from build123d import *

# Parameters (mm, degrees)
F0_R     = 11.0109
F0_R_2   = 3.175
F1_DEPTH = 6.35


with BuildPart() as f1:
    # F0 (on Front) → F1 (new body)
    with BuildSketch(Plane.XZ):
        with BuildLine():
            ThreePointArc((12.3733379566, 24.60625), (13.8006652431, 28.0521228931), (14.2875, 31.75))
            ThreePointArc((14.2875, 31.75), (10.1027881362, 41.8527881362), (0, 46.0375))
            ThreePointArc((0, 46.0375), (-10.1027881362, 41.8527881362), (-14.2875, 31.75))
            ThreePointArc((-14.2875, 31.75), (-13.8006652431, 28.0521228931), (-12.3733379566, 24.60625))
            ThreePointArc((-12.3733379566, 24.60625), (0, 17.4625), (12.3733379566, 24.60625))
        make_face()
        with Locations((0, 31.75)):
            Circle(F0_R, mode=Mode.SUBTRACT)
        with BuildLine():
            ThreePointArc((-14.2875, 31.75), (-10.1027881362, 41.8527881362), (0, 46.0375))
            ThreePointArc((0, 46.0375), (-20.8568006936, 40.269983922), (-35.7872332561, 24.60625))
            ThreePointArc((-35.7872332561, 24.60625), (-26.2265027578, 31.7569329924), (-14.2875, 31.75))
        make_face()
        with BuildLine():
            ThreePointArc((10.6471746219, 11.2874452221), (10.1786438017, 18.1194292121), (12.3733379566, 24.60625))
            ThreePointArc((12.3733379566, 24.60625), (0, 17.4625), (-12.3733379566, 24.60625))
            ThreePointArc((-12.3733379566, 24.60625), (-10.2077366082, 18.3335066447), (-10.5388292946, 11.7057230006))
            ThreePointArc((-10.5388292946, 11.7057230006), (-10.3260856779, 10.8481793102), (-10.2344309309, 9.9694071925))
            ThreePointArc((-10.2344309309, 9.9694071925), (0.1150101412, 14.2870370937), (10.3936009423, 9.8033522686))
            ThreePointArc((10.3936009423, 9.8033522686), (10.4762468955, 10.5529407036), (10.6471746219, 11.2874452221))
        make_face()
        with BuildLine():
            ThreePointArc((23.0855388403, 9.4834715128), (17.6469627848, 15.7677221756), (10.6471746219, 11.2874452221))
            ThreePointArc((10.6471746219, 11.2874452221), (11.3765560575, 9.1599013663), (12.3733379177, 7.1437500673))
            ThreePointArc((12.3733379177, 7.1437500673), (13.7532190864, 5.1015858399), (15.4068681354, 3.274032395))
            ThreePointArc((15.4068681354, 3.274032395), (20.7283724847, 4.5458830844), (23.0855388403, 9.4834715128))
        make_face()
        with Locations((16.7355388403, 9.4834715128)):
            Circle(F0_R_2, mode=Mode.SUBTRACT)
        with BuildLine():
            ThreePointArc((12.3733379177, 7.1437500673), (11.3765560575, 9.1599013663), (10.6471746219, 11.2874452221))
            ThreePointArc((10.6471746219, 11.2874452221), (10.4762468955, 10.5529407036), (10.3936009423, 9.8033522686))
            ThreePointArc((10.3936009423, 9.8033522686), (11.4608789903, 8.531172781), (12.3733379177, 7.1437500673))
        make_face()
        with BuildLine():
            ThreePointArc((-10.2344309309, 9.9694071925), (-10.3260856779, 10.8481793102), (-10.5388292946, 11.7057230006))
            ThreePointArc((-10.5388292946, 11.7057230006), (-11.2947124555, 9.359844254), (-12.3733379294, 7.1437500471))
            ThreePointArc((-12.3733379294, 7.1437500471), (-11.3918342591, 8.6231530466), (-10.2344309309, 9.9694071925))
        make_face()
        with BuildLine():
            ThreePointArc((-12.3733379294, 7.1437500471), (-11.2947124555, 9.359844254), (-10.5388292946, 11.7057230006))
            ThreePointArc((-10.5388292946, 11.7057230006), (-22.1188173057, 12.8583877354), (-15.0988016171, 3.57700109))
            ThreePointArc((-15.0988016171, 3.57700109), (-13.620985268, 5.2724359227), (-12.3733379294, 7.1437500471))
        make_face()
        with Locations((-16.5806966663, 9.7516660253)):
            Circle(F0_R_2, mode=Mode.SUBTRACT)
        with BuildLine():
            ThreePointArc((15.4068681354, 3.274032395), (13.7532190864, 5.1015858399), (12.3733379177, 7.1437500673))
            ThreePointArc((12.3733379177, 7.1437500673), (13.1637867029, 5.5540414017), (13.7509753549, 3.8785735832))
            ThreePointArc((13.7509753549, 3.8785735832), (14.5578417064, 3.5185628636), (15.4068681354, 3.274032395))
        make_face()
        with BuildLine():
            ThreePointArc((-13.686752578, 4.0994463185), (-13.1186518214, 5.6598260255), (-12.3733379294, 7.1437500471))
            ThreePointArc((-12.3733379294, 7.1437500471), (-13.620985268, 5.2724359227), (-15.0988016171, 3.57700109))
            ThreePointArc((-15.0988016171, 3.57700109), (-14.3772381817, 3.796225596), (-13.686752578, 4.0994463185))
        make_face()
        with BuildLine():
            ThreePointArc((-13.686752578, 4.0994463185), (-14.3772381817, 3.796225596), (-15.0988016171, 3.57700109))
            ThreePointArc((-15.0988016171, 3.57700109), (-20.7812079006, -0.2447504977), (-27.4963065702, -1.5875))
            ThreePointArc((-27.4963065702, -1.5875), (-17.393518434, -5.7722118638), (-13.2088065702, -15.875))
            ThreePointArc((-13.2088065702, -15.875), (-13.6956413271, -19.5728771069), (-15.1229686136, -23.01875))
            ThreePointArc((-15.1229686136, -23.01875), (-10.7734141907, -18.0069125403), (-4.8680388409, -14.9797553955))
            ThreePointArc((-4.8680388409, -14.9797553955), (-4.2317560285, -14.3667421738), (-3.5165444239, -13.8479807757))
            ThreePointArc((-3.5165444239, -13.8479807757), (-12.4304421386, -7.0439168429), (-13.686752578, 4.0994463185))
        make_face()
        with BuildLine():
            ThreePointArc((15.4068681354, 3.274032395), (14.5578417064, 3.5185628636), (13.7509753549, 3.8785735832))
            ThreePointArc((13.7509753549, 3.8785735832), (14.1527332454, 1.9577532873), (14.2875, 0))
            ThreePointArc((14.2875, 0), (11.2067738499, -8.8623290464), (3.2931516357, -13.9027985871))
            ThreePointArc((3.2931516357, -13.9027985871), (3.9009912862, -14.3491662996), (4.4516269953, -14.8644463122))
            ThreePointArc((4.4516269953, -14.8644463122), (10.6025640989, -17.8746787144), (15.1229686136, -23.01875))
            ThreePointArc((15.1229686136, -23.01875), (15.1229686136, -8.73125), (27.4963065702, -1.5875))
            ThreePointArc((27.4963065702, -1.5875), (20.9811507989, -0.3265941045), (15.4068681354, 3.274032395))
        make_face()
        with BuildLine():
            ThreePointArc((-13.2088065702, -15.875), (-17.393518434, -5.7722118638), (-27.4963065702, -1.5875))
            ThreePointArc((-27.4963065702, -1.5875), (-39.8696445267, -8.73125), (-39.8696445267, -23.01875))
            ThreePointArc((-39.8696445267, -23.01875), (-31.1941836771, -29.6756652431), (-20.3525565702, -28.2483379566))
            ThreePointArc((-20.3525565702, -28.2483379566), (-17.393518434, -25.9777881362), (-15.1229686136, -23.01875))
            ThreePointArc((-15.1229686136, -23.01875), (-13.6956413271, -19.5728771069), (-13.2088065702, -15.875))
        make_face()
        with Locations((-27.4963065702, -15.875)):
            Circle(F0_R, mode=Mode.SUBTRACT)
        with BuildLine():
            ThreePointArc((34.6400565702, -3.5016620434), (31.1941836771, -2.0743347569), (27.4963065702, -1.5875))
            ThreePointArc((27.4963065702, -1.5875), (15.1229686136, -8.73125), (15.1229686136, -23.01875))
            ThreePointArc((15.1229686136, -23.01875), (27.4963065702, -30.1625), (39.8696445267, -23.01875))
            ThreePointArc((39.8696445267, -23.01875), (41.2969718133, -19.5728771069), (41.7838065702, -15.875))
            ThreePointArc((41.7838065702, -15.875), (39.8696445267, -8.73125), (34.6400565702, -3.5016620434))
        make_face()
        with Locations((27.4963065702, -15.875)):
            Circle(F0_R, mode=Mode.SUBTRACT)
        with BuildLine():
            ThreePointArc((-5.5e-09, -14.2875), (-1.7719524453, -14.1771943903), (-3.5165444239, -13.8479807757))
            ThreePointArc((-3.5165444239, -13.8479807757), (-4.2317560285, -14.3667421738), (-4.8680388409, -14.9797553955))
            ThreePointArc((-4.8680388409, -14.9797553955), (-2.4585066475, -14.4614300385), (-5.5e-09, -14.2875))
        make_face()
        with BuildLine():
            ThreePointArc((-20.3525565702, -28.2483379566), (-31.1941836771, -29.6756652431), (-39.8696445267, -23.01875))
            ThreePointArc((-39.8696445267, -23.01875), (-24.4464287396, -38.1975112033), (-3.4160209638, -43.2957781309))
            ThreePointArc((-3.4160209638, -43.2957781309), (-14.3890593388, -38.5912841369), (-20.3525565702, -28.2483379566))
        make_face()
        with BuildLine():
            ThreePointArc((4.4516269953, -14.8644463122), (3.9009912862, -14.3491662996), (3.2931516357, -13.9027985871))
            ThreePointArc((3.2931516357, -13.9027985871), (1.6577728159, -14.1909987506), (-5.5e-09, -14.2875))
            ThreePointArc((-5.5e-09, -14.2875), (2.2444292093, -14.4323372312), (4.4516269953, -14.8644463122))
        make_face()
        with BuildLine():
            ThreePointArc((39.2032542199, 18.6895281309), (40.6155620966, 6.8343511445), (34.6400565702, -3.5016620434))
            ThreePointArc((34.6400565702, -3.5016620434), (39.8696445267, -8.73125), (41.7838065702, -15.875))
            ThreePointArc((41.7838065702, -15.875), (41.2969718133, -19.5728771069), (39.8696445267, -23.01875))
            ThreePointArc((39.8696445267, -23.01875), (45.3032294332, -2.0724727187), (39.2032542199, 18.6895281309))
        make_face()
        with BuildLine():
            ThreePointArc((4.4516269953, -14.8644463122), (2.2444292093, -14.4323372312), (-5.5e-09, -14.2875))
            ThreePointArc((-5.5e-09, -14.2875), (-2.4585066475, -14.4614300385), (-4.8680388409, -14.9797553955))
            ThreePointArc((-4.8680388409, -14.9797553955), (-2.4345023642, -25.1618271215), (6.195157826, -19.2351375381))
            ThreePointArc((6.195157826, -19.2351375381), (5.743190516, -16.8823284962), (4.4516269953, -14.8644463122))
        make_face()
        with Locations((-0.154842174, -19.2351375381)):
            Circle(F0_R_2, mode=Mode.SUBTRACT)
        with BuildLine():
            ThreePointArc((13.7509753549, 3.8785735832), (11.2108978898, 6.3528418048), (10.3936009423, 9.8033522686))
            ThreePointArc((10.3936009423, 9.8033522686), (0.1150101412, 14.2870370937), (-10.2344309309, 9.9694071925))
            ThreePointArc((-10.2344309309, 9.9694071925), (-10.2316303011, 9.8605526184), (-10.2306966663, 9.7516660253))
            ThreePointArc((-10.2306966663, 9.7516660253), (-11.1631767097, 6.4391175321), (-13.686752578, 4.0994463185))
            ThreePointArc((-13.686752578, 4.0994463185), (-12.4304421386, -7.0439168429), (-3.5165444239, -13.8479807757))
            ThreePointArc((-3.5165444239, -13.8479807757), (-0.1037265557, -12.8853432742), (3.2931516357, -13.9027985871))
            ThreePointArc((3.2931516357, -13.9027985871), (11.2067738499, -8.8623290464), (14.2875, 0))
            ThreePointArc((14.2875, 0), (14.1527332454, 1.9577532873), (13.7509753549, 3.8785735832))
        make_face()
        Circle(F0_R, mode=Mode.SUBTRACT)
        with BuildLine():
            ThreePointArc((3.2931516357, -13.9027985871), (-0.1037265557, -12.8853432742), (-3.5165444239, -13.8479807757))
            ThreePointArc((-3.5165444239, -13.8479807757), (-1.7719524453, -14.1771943903), (-5.5e-09, -14.2875))
            ThreePointArc((-5.5e-09, -14.2875), (1.6577728159, -14.1909987506), (3.2931516357, -13.9027985871))
        make_face()
        with BuildLine():
            ThreePointArc((-10.2344309309, 9.9694071925), (-11.3918342591, 8.6231530466), (-12.3733379294, 7.1437500471))
            ThreePointArc((-12.3733379294, 7.1437500471), (-13.1186518214, 5.6598260255), (-13.686752578, 4.0994463185))
            ThreePointArc((-13.686752578, 4.0994463185), (-11.1631767097, 6.4391175321), (-10.2306966663, 9.7516660253))
            ThreePointArc((-10.2306966663, 9.7516660253), (-10.2316303011, 9.8605526184), (-10.2344309309, 9.9694071925))
        make_face()
        with BuildLine():
            ThreePointArc((13.7509753549, 3.8785735832), (13.1637867029, 5.5540414017), (12.3733379177, 7.1437500673))
            ThreePointArc((12.3733379177, 7.1437500673), (11.4608789903, 8.531172781), (10.3936009423, 9.8033522686))
            ThreePointArc((10.3936009423, 9.8033522686), (11.2108978898, 6.3528418048), (13.7509753549, 3.8785735832))
        make_face()
    extrude(amount=F1_DEPTH)


solid = f1.part
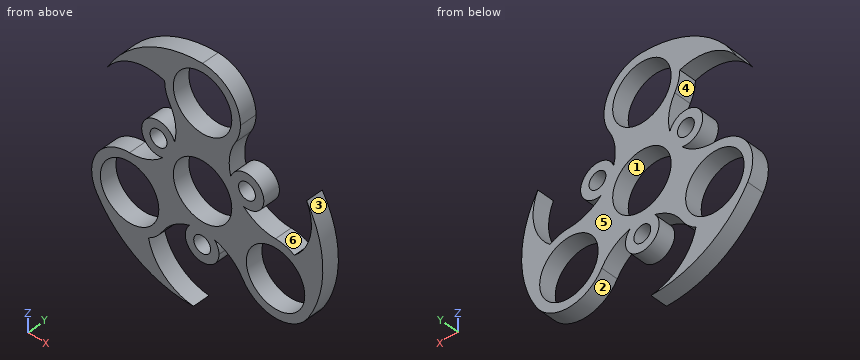
Verification items for the finished model (mm, model axes). Face numbers are marked on the shaded views. A direction names the side the tool comes from. Give positions to 0.01 mm unless a question says otherwise; leave off trailing zeros. Loops run counter-clockwise (first coordinate to the right, second up) from the corner with the lowest first, then second, coordinate; pieces in that order, holes last. Notation, with made-up numbers: (-14.75, -22) - (-8.75, -22) arc R14 ccw to (-8.75, 0) - close; hole circle Ø7 at (68.5, 10.25). An arc over 180 degrees is marked (long way). Write item = value, one per line. Start each with the question number.
Q1. Depth check by flat-ended pin: P1, Ø2, axis at y = -1.5, z = -8.5, coming from the +X side; P2, Ø17.5, axis at x = -27.5, z = -15.88, coming from the -Y side; P3, Ø3, axis at x = 3.5, y = -3.5, coming from the -Z side. Enter the tip coordinate at first touch or a pass-through.
Q2. Cross-section at B-B, the plane z = 0. Enter the section's corners in (x, y), and give its area (3 significant figures).
Q3. Tool access check on the marked faces 4, 5 and 6. Record the directions out of +Z, -Z, +X, -X, +Y, -Y that give a thin tool (end or side, any length) a straight path to the whole face; none if there is none.
Q4. Cross-section at D-D, the plane y = -5. State how many separate pieces and enclosed holes the cut face has, and give its area (3 significant figures).
Q5. Mould release check, pull along Z, two halves, no side actions. Record for the marked faces 1, 2 and 3: released by +Z, released by -Z, zero draft, split by the parting line, or undercut.
Q6. Cross-section at A-A, the plane x = -18. Enter the section's corners in (y, z).
Q7. Cross-section at C-C, the plane x = 1. Enter the section's corners in (y, z), and give its area (3 significant figures).
Q8. Thickness scan on line 1 (X direction, y = -1, z = -22); line 2 (X direction, y = -0.5, z = -7.5); line 3 (X direction, y = -5, z = -16.5). Record the ranges inside material, lowest first.
Answer key:
q1.P1 = 45.03
q1.P2 = through
q1.P3 = -25.21
q2.outline = (-20.22, -6.35) - (-11.01, -6.35) - (-11.01, 0) - (-20.22, 0) - close; (11.01, -6.35) - (20.22, -6.35) - (20.22, 0) - (11.01, 0) - close; (37.72, -6.35) - (45.22, -6.35) - (45.22, 0) - (37.72, 0) - close
q2.area = 165 mm^2
q3.face_4 = +Y, -Y
q3.face_5 = +Z, -Z, +X, -X, +Y
q3.face_6 = +Z, +Y, -Y
q4.separate_pieces = 1
q4.enclosed_holes = 7
q4.area = 2,120 mm^2
q5.face_1 = undercut
q5.face_2 = released by -Z
q5.face_3 = split by the parting line
q6.outline = (-6.35, -41.08) - (0, -41.08) - (0, -34.26) - (-6.35, -34.26) - close; (-6.35, -26.55) - (0, -26.55) - (0, -21.45) - (-6.35, -21.45) - close; (-6.35, -10.3) - (0, -10.3) - (0, 1.22) - (-6.35, 1.22) - close; (-6.35, 3.56) - (0, 3.56) - (0, 6.91) - (-6.35, 6.91) - close; (-6.35, 12.59) - (0, 12.59) - (0, 15.94) - (-6.35, 15.94) - close; (-6.35, 32.58) - (0, 32.58) - (0, 41.83) - (-6.35, 41.83) - close
q7.outline = (-6.35, -25.48) - (0, -25.48) - (0, -22.19) - (-6.35, -22.19) - close; (-6.35, -16.28) - (0, -16.28) - (0, -10.97) - (-6.35, -10.97) - close; (-6.35, 10.97) - (0, 10.97) - (0, 20.78) - (-6.35, 20.78) - close; (-6.35, 42.72) - (0, 42.72) - (0, 46) - (-6.35, 46) - close
q7.area = 138 mm^2
q8.line_1 = -40.4 to -36.65, -18.35 to -14.49, -5.87 to -1.72, 1.41 to 5.56, 14.49 to 18.35, 36.65 to 40.44
q8.line_2 = -39.07 to -34.64, -20.35 to -8.06, 8.06 to 20.35, 34.64 to 45.03
q8.line_3 = -41.77 to -38.49, -16.5 to -8.51, -5.89 to -1.77, 1.46 to 5.58, 8.51 to 16.5, 38.49 to 42.9
